Here's how the part is built. I have some questions about the finished solid (model axes, mm). A direction names the side the tool comes from. Coordinates: 2 decimals unless noted, no trailing zeros. Loops run counter-clockwise (first coordinate to the right, second up) from the corner with the lowest first, then second, coordinate; pieces in that order, holes last. Notation, with made-up numbers: (34.5, 68) - (54.5, 68) arc R21 cw to (54.5, 74) - close; hole circle Ø3 at (84, 21.5). An arc over 180 degrees is marked (long way). Use a Markdown table: item, result.
```python
from build123d import *

# Parameters (mm, degrees)
SKETCH004_W  = 48
SKETCH004_H  = 43
PAD012_DEPTH = 60
SKETCH003_W  = 50
SKETCH003_H  = 45
PAD011_DEPTH = 60


with BuildPart() as body004:
    # Sketch004 → Pad012 (new body)
    with BuildSketch(Plane.XY.offset(-39)):
        Rectangle(SKETCH004_W, SKETCH004_H)
    extrude(amount=PAD012_DEPTH)


with BuildPart() as body004_1:
    # Body004 placement: moved
    add(body004.part.moved(Location((0, -37.9, -17))))


with BuildPart() as cut:
    # Sketch003 → Pad011 (new body)
    with BuildSketch(Plane.XY.offset(-40)):
        Rectangle(SKETCH003_W, SKETCH003_H)
    extrude(amount=PAD011_DEPTH)


with BuildPart() as cut_1:
    # Body003 placement: moved
    add(cut.part.moved(Location((0, -37.9, -18))))

    # Cut: cut Body004
    add(body004_1.part, mode=Mode.SUBTRACT)


solid = cut_1.part
```
Q1. Which directions (+Z, -Z, +X, -X, +Y, -Y) give clear straight access to the entire face, cutting with the end or side of a thin tool? Please do faces 4 (the face through (-24.2, -37.8, 2)), 5 (the face through (24, -38, -27)).
Check values:
| item | result |
|---|---|
| face 4 | +Z, +X, -X, +Y, -Y |
| face 5 | +Z |
Q2. I want a section at C-C, the plane x = -10. Write out the boundary of the cut face in (y, z), then the cut area to 3 significant figures.
Check values:
| item | result |
|---|---|
| outline | (-60.4, -58) - (-15.4, -58) - (-15.4, 2) - (-16.4, 2) - (-16.4, -56) - (-59.4, -56) - (-59.4, 2) - (-60.4, 2) - close |
| area | 206 mm^2 |
Q3. Please list where these lines run through material, in increasing order: L1, parallel to X at y = -54, z = -41.5; L2, parallel to Y at x = 14.5, z = -29; L3, parallel to Z at x = 9, y = -27. Write a range as from..to.
Check values:
| item | result |
|---|---|
| L1 | -25..-24, 24..25 |
| L2 | -60.4..-59.4, -16.4..-15.4 |
| L3 | -58..-56 |
Q4. I want a section at B-B, the plane y = -26. Write out the boundary of the cut face in (x, z).
Check values:
| item | result |
|---|---|
| outline | (-25, -58) - (25, -58) - (25, 2) - (24, 2) - (24, -56) - (-24, -56) - (-24, 2) - (-25, 2) - close |
Q5. Will this pin go through, and if not, where does the flat tip stop? P1, Ø12, axis at x = -2, y = -24, coming from the +Z side.
Check values:
| item | result |
|---|---|
| P1 | z = -56 |
Q6. I want a section at A-A, the plane z = -37.5. Write out the boundary of the cut face in (x, y), then the cut area to 3 significant figures.
Check values:
| item | result |
|---|---|
| outline | (-25, -60.4) - (25, -60.4) - (25, -15.4) - (-25, -15.4) - close; hole (-24, -59.4) - (24, -59.4) - (24, -16.4) - (-24, -16.4) - close |
| area | 186 mm^2 |
Q7. If we mould it in two halves opening along Y, with no side actions, what happens to faces 1 (the face through (0, -60.4, -28)), 2 (the face through (25, -38, -28)), 3 (the face through (-24, -38, -27))? For each: pulls with the +Y half, pulls with the -Y half, needs draft (parallel to the pull), parting line crosses it, or undercut.
Check values:
| item | result |
|---|---|
| face 1 | pulls with the -Y half |
| face 2 | needs draft |
| face 3 | undercut |
